```python
from build123d import *

# Parameters (mm, degrees)
SKETCH_3_R          = 25
EXTRUDE_1_DEPTH     = 340
SKETCH_6_R          = 45
EXTRUDE_2_DEPTH     = 10
EXTRUDE_START       = 10
SKETCH_7_R          = 45
EXTRUDE_3_DEPTH     = 10
SKETCH_4_R          = 20
CUT_EXTRUDE_1_DEPTH = 366.581728209
SKETCH_8_W          = 40.591982286
SKETCH_8_H          = 75.225313462
CUT_EXTRUDE_2_DEPTH = 366.581728209
SKETCH_9_W          = 20
SKETCH_9_H          = 290
CUT_EXTRUDE_3_DEPTH = 357.405667744
M6X1_0_1_D          = 5
FILLET_1_R          = 5
SKETCH_12_R         = 2.55
CUT_EXTRUDE_4_DEPTH = 364.641702853
SKETCH_13_W         = 245.746793121
SKETCH_13_H         = 335.021693113
CUT_EXTRUDE_5_DEPTH = 180
CUT_EXTRUDE_7_DEPTH = 30
EXTRUDE_4_DEPTH     = 10
FILLET_5_R          = 0.5
FILLET_6_R          = 0.5


with BuildPart() as part:
    # 草图3 → 凸台-拉伸1 (new body)
    with BuildSketch(Plane(origin=(0, 0, 0), x_dir=(1, 0, 0), z_dir=(0, 1, 0))):
        with Locations(Location((0, 0, 0), (0, 0, 270))):
            Circle(SKETCH_3_R)
    extrude(amount=EXTRUDE_1_DEPTH)

    # 草图6 → 凸台-拉伸2 (add)
    with BuildSketch(Plane.XZ):
        with Locations(Location((0, 0, 0), (0, 0, 270))):
            Circle(SKETCH_6_R)
    extrude(amount=EXTRUDE_2_DEPTH)

    # 草图7 → 凸台-拉伸3 (add)
    with BuildSketch(Plane(origin=(0, 340, 0), x_dir=(1, 0, 0), z_dir=(0, 1, 0)).offset(EXTRUDE_START)):
        with Locations(Location((0, 0, 0), (0, 0, 90))):
            Circle(SKETCH_7_R)
    extrude(amount=-EXTRUDE_3_DEPTH)

    # 草图4 → 切除-拉伸1 (cut, through all)
    with BuildSketch(Plane.XZ.offset(10)):
        with Locations(Location((0, 0, 0), (0, 0, 270))):
            Circle(SKETCH_4_R)
    extrude(amount=-CUT_EXTRUDE_1_DEPTH, mode=Mode.SUBTRACT)

    # 草图8 → 切除-拉伸2 (cut, through all)
    with BuildSketch(Plane(origin=(0, 350, 0), x_dir=(1, 0, 0), z_dir=(0, 1, 0))):
        with Locations((45, 0)):
            Rectangle(SKETCH_8_W, SKETCH_8_H)
    cut_extrude_2 = extrude(amount=-CUT_EXTRUDE_2_DEPTH, mode=Mode.SUBTRACT)

    # 草图9 → 切除-拉伸3 (cut, through all)
    with BuildSketch(Plane(origin=(-25.295991143, 0, 0), x_dir=(0, 0, -1), z_dir=(1, 0, 0))):
        with Locations((0, 170)):
            Rectangle(SKETCH_9_W, SKETCH_9_H)
    extrude(amount=CUT_EXTRUDE_3_DEPTH, mode=Mode.SUBTRACT)

    # M6x1.0 螺纹孔1 (through all)
    with Locations(Plane(origin=(0, 350, 0), x_dir=(1, 0, 0), z_dir=(0, 1, 0))):
        with Locations((0, -35), (0, 35)):
            Hole(M6X1_0_1_D / 2)

    # 镜向1: 切除-拉伸2 across plane
    add(cut_extrude_2.mirror(Plane(origin=(0, 0, 0), x_dir=(0, 0, 1), z_dir=(1, 0, 0))), mode=Mode.SUBTRACT)

    # 圆角1
    fillet_1_edges = [part.edges().sort_by_distance(p)[0] for p in [
        (-24.704008857, -5, -37.612656731),
        (-24.704008857, 345, -37.612656731),
        (-24.704008857, -5, 37.612656731),
        (-24.704008857, 345, 37.612656731),
        (24.704008857, -5, 37.612656731),
        (24.704008857, 345, 37.612656731),
        (24.704008857, -5, -37.612656731),
        (24.704008857, 345, -37.612656731),
    ]]
    fillet(fillet_1_edges, radius=FILLET_1_R)

    # 草图12 → 切除-拉伸4 (cut, through all)
    with BuildSketch(Plane(origin=(0, 350, 0), x_dir=(1, 0, 0), z_dir=(0, 1, 0))):
        with Locations(Location((0, 35, 0), (0, 0, 270))):
            Circle(SKETCH_12_R)
        with Locations(Location((0, -35, 0), (0, 0, 270))):
            Circle(SKETCH_12_R)
    extrude(amount=-CUT_EXTRUDE_4_DEPTH, mode=Mode.SUBTRACT)

    # 草图13 → 切除-拉伸5 (cut)
    with BuildSketch(Plane.XZ.offset(10)):
        with Locations((-21.384575648, -11.685004811)):
            Rectangle(SKETCH_13_W, SKETCH_13_H)
    extrude(amount=-CUT_EXTRUDE_5_DEPTH, mode=Mode.SUBTRACT)

    # 草图16 → 切除-拉伸7 (cut)
    with BuildSketch(Plane.XZ.offset(-170)):
        with BuildLine():
            ThreePointArc((-20.321384852, -11.732557014), (-17.43797807, -15.701225978), (-13.79244797, -18.983676024))
            ThreePointArc((-13.79244797, -18.983676024), (-12.395645723, -18.762444282), (-12.616877465, -17.365642036))
            ThreePointArc((-12.616877465, -17.365642036), (-15.951688419, -14.362964766), (-18.589334044, -10.732557014))
            ThreePointArc((-18.589334044, -10.732557014), (-19.955359448, -10.366531611), (-20.321384852, -11.732557014))
        make_face()
        with BuildLine():
            ThreePointArc((13.79244797, -18.983676024), (17.43797807, -15.701225978), (20.321384852, -11.732557014))
            ThreePointArc((20.321384852, -11.732557014), (19.955359448, -10.366531611), (18.589334044, -10.732557014))
            ThreePointArc((18.589334044, -10.732557014), (15.951688419, -14.362964766), (12.616877465, -17.365642036))
            ThreePointArc((12.616877465, -17.365642036), (12.395645723, -18.762444282), (13.79244797, -18.983676024))
        make_face()
    extrude(amount=-CUT_EXTRUDE_7_DEPTH, mode=Mode.SUBTRACT)

    # 草图17 → 凸台-拉伸4 (add)
    with BuildSketch(Plane.XZ.offset(-170)):
        with BuildLine():
            ThreePointArc((20.148179771, 11.632557014), (17.289349105, 15.567399857), (13.674890919, 18.821872625))
            ThreePointArc((13.674890919, 18.821872625), (12.557449122, 18.644887232), (12.734434515, 17.527445434))
            ThreePointArc((12.734434515, 17.527445434), (16.100317384, 14.496790887), (18.762539125, 10.832557014))
            ThreePointArc((18.762539125, 10.832557014), (19.855359448, 10.539736691), (20.148179771, 11.632557014))
        make_face()
        with BuildLine():
            ThreePointArc((-13.674890919, 18.821872625), (-17.289349105, 15.567399857), (-20.148179771, 11.632557014))
            ThreePointArc((-20.148179771, 11.632557014), (-19.855359448, 10.539736691), (-18.762539125, 10.832557014))
            ThreePointArc((-18.762539125, 10.832557014), (-16.100317384, 14.496790887), (-12.734434515, 17.527445434))
            ThreePointArc((-12.734434515, 17.527445434), (-12.557449122, 18.644887232), (-13.674890919, 18.821872625))
        make_face()
    extrude(amount=EXTRUDE_4_DEPTH)

    # 圆角5
    fillet_5_edges = [part.edges().sort_by_distance(p)[0] for p in [
        (-12.557449122, 160, 18.644887232),
        (-17.289349105, 160, 15.567399857),
        (-19.855359448, 160, 10.539736691),
        (-16.100317384, 160, 14.496790887),
    ]]
    fillet(fillet_5_edges, radius=FILLET_5_R)

    # 圆角6
    fillet_6_edges = [part.edges().sort_by_distance(p)[0] for p in [
        (19.855359448, 160, 10.539736691),
        (17.289349105, 160, 15.567399857),
        (12.557449122, 160, 18.644887232),
        (16.100317384, 160, 14.496790887),
    ]]
    fillet(fillet_6_edges, radius=FILLET_6_R)


solid = part.part
```
The listing builds one solid part. Answer for the finished solid, in the listing's coordinates (mm). A direction names the side the tool comes from. Round coordinates to 2 decimals unless told otherwise and drop trailing zeros. Loops run counter-clockwise (first coordinate to the right, second up) from the corner with the lowest first, then second, coordinate; pieces in that order, holes last. Notation, with made-up numbers: (29, 34.5) - (61, 34.5) arc R31 ccw to (61, 72.5) - close; hole circle Ø9 at (-14, 10.25). An arc over 180 degrees is marked (long way). Return JSON: item names as keys, results as strings. Group by question number.
1. Each of these flat-tipped pins is pushed along its axis until it touches: P1, Ø6, axis at y = 199.5, z = 12, coming from the +X side; P2, Ø3, axis at x = 21.5, y = 207.5, coming from the +Z side; P3, Ø8, axis at x = -15.5, z = 6, coming from the -Y side. Where does it stop, or does it pass through?
2. The part is cut by section B-B on z = 0. Determine the outline of the cut face in (x, y).
3. The part is cut by section A-A on y = 236. Determine the outline of the cut face in (x, z), then the cut area to 3 significant figures.
4. The part is cut by section C-C on x = 7. Determine the outline of the cut face in (y, z) (3 decimals), then the cut area to 3 significant figures.
5. The mould has two halves that part along Z. Classify faces 4 (the cylindrical face through (0, 345, 45)), 5 (the cylindrical face through (16.864, 258.74, -10.752)), 6 (the cylindrical face through (-24.04, 344.93, -37.3)): pulls with the +Z half, pulls with the -Z half, needs draft (parallel to the pull), parting line crosses it, or undercut.
6. Consider probe 1 along X at (y, z) = (261, -14.5); probe 2 along X at (y, z) = (344, -35); probe 3 along Y at (x, z) = (6, -33). Determine where each line is inside the solid, lowest interval first.
7. Which of the six approach directions +Z, -Z, +X, -X, +Y, -Y give full straight-line access (tool end or side, diameter ignored) to faces 1 (the flat face through (0, 340, -29)), 2 (the flat face through (-20, 241, -10)), 3 (the flat face through (-0.1, 170, 20.3))?
8. The part is cut by section D-D on y = 334.5. Determine the outline of the cut face in (x, z), then the cut area to 3 significant figures.
Resolved:
{
 "1": {"P1": "stops at x = 22.91", "P2": "stops at z = 15", "P3": "stops at y = 315"},
 "2": {"outline": "(-24.7, 315) - (-20, 315) - (-20, 350) - (-24.7, 350) - close; (20, 315) - (24.7, 315) - (24.7, 350) - (20, 350) - close"},
 "3": {"outline": "(-22.91, -10) arc R25 ccw to (22.91, -10) - (17.32, -10) arc R20 cw to (-17.32, -10) - close; (-22.91, 10) - (-17.32, 10) arc R20 cw to (17.32, 10) - (22.91, 10) arc R25 ccw to start", "area": "499 mm²"},
 "4": {"outline": "(170, -24) - (340, -24) - (340, -44.452) - (350, -44.452) - (350, -18.735) - (170, -18.735) - close; (170, 18.735) - (350, 18.735) - (350, 44.452) - (340, 44.452) - (340, 24) - (170, 24) - close", "area": "2,300 mm²"},
 "5": {"face 4": "pulls with the +Z half", "face 5": "undercut", "face 6": "pulls with the -Z half"},
 "6": {"probe 1": "x = -20.37 to -13.77, 13.77 to 20.37", "probe 2": "x = -24.7 to -2.55, 2.55 to 24.7", "probe 3": "y = 340 to 350"},
 "7": {"face 1": "-Z, -Y", "face 2": "+X, -X, -Y", "face 3": "-Y"},
 "8": {"outline": "(-24.7, -3.84) arc R25 ccw to (24.7, -3.84) - (24.7, 3.84) arc R25 ccw to (-24.7, 3.84) - close; hole circle Ø40 at (0, 0)", "area": "704 mm²"}
}
